Geometry: final body of the model. Coordinates: model frame, mm. Face numbers are marked on the shaded views. Round coordinates to 2 decimals unless told otherwise and drop trailing zeros. Write each loop counter-clockwise with the first axis right and the second up, starting at its lowest first coordinate (ties: lowest second). Pieces come first, ordered by that corner, then holes.
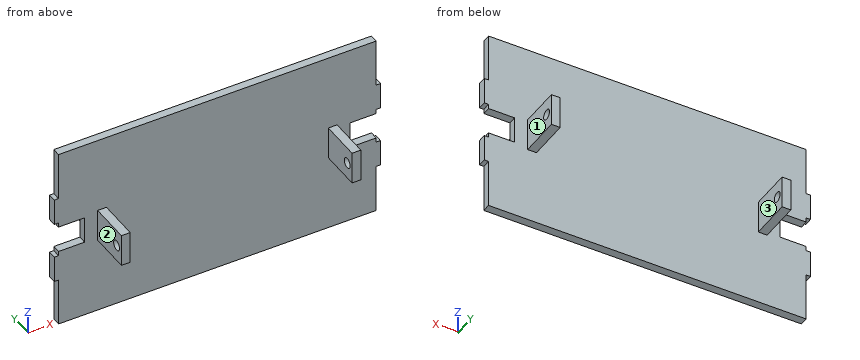
from build123d import *

# Parameters (mm, degrees)
BOSS_EXTRUDE1_DEPTH     = 3.175
SKETCH2_W               = 6.858
SKETCH2_H               = 25.4
BOSS_EXTRUDE2_DEPTH     = 35.052
CUT_EXTRUDE1_DEPTH      = 235.445990215
CUT_EXTRUDE1_DEPTH_BACK = 235.445990215
SKETCH3_R               = 3.937


with BuildPart() as part:
    # Sketch1 → Boss-Extrude1 (new, symmetric)
    with BuildSketch(Plane(origin=(0, 0, 0), x_dir=(1, 0, 0), z_dir=(0, 1, 0))):
        Polygon((123.698, -72.39), (-123.698, -72.39), (-123.698, -34.798), (-127, -34.798), (-127, -13.97), (-123.698, -13.97), (-123.698, -10.414), (-103.378, -10.414), (-103.378, 10.414), (-123.698, 10.414), (-123.698, 13.97), (-127, 13.97), (-127, 34.798), (-123.698, 34.798), (-123.698, 72.39), (123.698, 72.39), (123.698, 34.798), (127, 34.798), (127, 13.97), (123.698, 13.97), (123.698, 10.414), (103.378, 10.414), (103.378, -10.414), (123.698, -10.414), (123.698, -13.97), (127, -13.97), (127, -34.798), (123.698, -34.798), align=None)
    extrude(amount=BOSS_EXTRUDE1_DEPTH, both=True)

    # Sketch2 → Boss-Extrude2 (add, symmetric)
    with BuildSketch(Plane(origin=(0, 0, 0), x_dir=(1, 0, 0), z_dir=(0, 1, 0))):
        with Locations((89.789, 0)):
            Rectangle(SKETCH2_W, SKETCH2_H)
        with Locations((-89.789, 0)):
            Rectangle(SKETCH2_W, SKETCH2_H)
    extrude(amount=BOSS_EXTRUDE2_DEPTH, both=True)

    # Sketch3 → Cut-Extrude1 (cut, two sides: drawn at the far end of the back side and taken through both)
    with BuildSketch(Plane.ZY.offset(93.218).offset(-CUT_EXTRUDE1_DEPTH_BACK)):
        with Locations((0, 28.575)):
            Circle(SKETCH3_R)
        with Locations((0, -28.575)):
            Circle(SKETCH3_R)
    extrude(amount=CUT_EXTRUDE1_DEPTH + CUT_EXTRUDE1_DEPTH_BACK, mode=Mode.SUBTRACT)


solid = part.part
1) Line query: probe 1 along Y at (x, z) = (-89, 0); probe 2 along X at (y, z) = (11.5, 12); probe 3 along Z at (x, y) = (-105.5, 0). Output: solid intervals per line, ascending.
2) Section C-C on x = 17. Output: boundary loops of the cut face in (y, z) (3 decimals), plus the area to 3 significant figures.
3) First-contact query: P1, Ø7.5, axis at y = -17, z = -4.5, coming from the +X side; P2, Ø1, axis at x = -41.5, z = -3, coming from the -Y side (3 decimals); P3, Ø3.5, axis at x = -91, y = 17.5, coming from the +Z side; P4, Ø6.5, axis at y = -28.575, z = 0, coming from the -X side. Flat tips, straight axial feed; report the tip coordinate or a pass-through.
4) Section D-D on z = -51. Output: boundary loops of the cut face in (x, y) (3 decimals), plus the area to 3 significant figures.
5) Section B-B on z = 0. State how many separate pieces and enclosed holes the cut face has, plus the area to 3 significant figures.
6) Draft query along X for the marked faces 1, 2 and 3. Return one class per face: pulls with the +X half, pulls with the -X half, needs draft (parallel to the pull), parting line crosses it, or undercut.
7) Section A-A on y = 10. Output: boundary loops of the cut face in (x, z), plus the area to 3 significant figures.
Filled in:
1. probe 1: y = -35.05 to -32.51, -24.64 to 24.64, 32.51 to 35.05
1. probe 2: x = -93.22 to -86.36, 86.36 to 93.22
1. probe 3: z = -72.39 to -10.41, 10.41 to 72.39
2. outline: (-3.175, -72.39) - (3.175, -72.39) - (3.175, 72.39) - (-3.175, 72.39) - close
2. area: 919 mm2
3. P1: stops at x = 93.22
3. P2: stops at y = -3.175
3. P3: stops at z = 12.7
3. P4: passes through
4. outline: (-123.698, -3.175) - (123.698, -3.175) - (123.698, 3.175) - (-123.698, 3.175) - close
4. area: 1,570 mm2
5. separate pieces: 5
5. enclosed holes: 0
5. area: 1,970 mm2
6. face 1: pulls with the +X half
6. face 2: pulls with the -X half
6. face 3: undercut
7. outline: (-93.22, -12.7) - (-86.36, -12.7) - (-86.36, 12.7) - (-93.22, 12.7) - close; (86.36, -12.7) - (93.22, -12.7) - (93.22, 12.7) - (86.36, 12.7) - close
7. area: 348 mm2
